Design review of the part built by this model. Coordinates are the model's own, in mm. Coordinates: 2 decimals unless noted, no trailing zeros. Loops run counter-clockwise (first coordinate to the right, second up) from the corner with the lowest first, then second, coordinate; pieces in that order, holes last. Notation, with made-up numbers: (71, 9.25) -> (97, 9.25) arc R21 cw to (97, 19.25) -> close; hole circle Ø4 at (76.25, 58.25). An arc over 180 degrees is marked (long way). Use a Markdown table: item, result. Add a question column.
Q1. For probe 1 along Y at (x, z) = (35, 2.5); probe 2 along Y at (x, z) = (27, 0.75), list the stretches that pass through material, from the lowest coordinate up.
Q2. Clearance check with flat-ended pins moving along their axes: pin 1 Ø3 at (x, y) = (272.72, 11.25) entering from -Z; pin 2 Ø6 at (x, y) = (154, 11.25) entering from +Z. State where each tip first meets the part, or that it passes through.
Q3. Take a section at A-A on z = 2. Write out the cut boundary in (x, y).
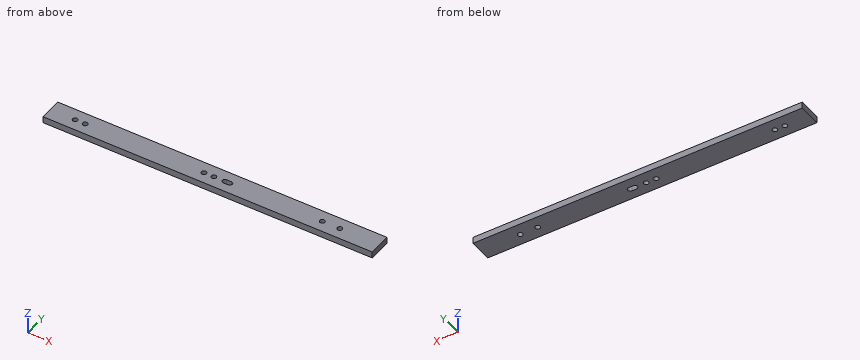
from build123d import *

# Parameters (mm, degrees)
SKETCH_W     = 330
SKETCH_H     = 23
PAD_DEPTH    = 6.5
SKETCH001_R  = 2.5
POCKET_DEPTH = 6.501


with BuildPart() as part:
    # Sketch → Pad (new body)
    with BuildSketch(Plane.XY):
        with Locations((165, 11.5)):
            Rectangle(SKETCH_W, SKETCH_H)
    extrude(amount=PAD_DEPTH)

    # Sketch001 (on Face6 of Pad) → Pocket (cut, through all)
    with BuildSketch(Plane.XY.offset(6.5)):
        with Locations((25, 11.25)):
            Circle(SKETCH001_R)
        with Locations((35, 11.25)):
            Circle(SKETCH001_R)
        with Locations((154, 11.25)):
            Circle(SKETCH001_R)
        with Locations((164, 11.25)):
            Circle(SKETCH001_R)
        with Locations((272.722137, 11.25)):
            Circle(SKETCH001_R)
        with Locations((290.250244, 11.25)):
            Circle(SKETCH001_R)
        with BuildLine():
            ThreePointArc((175, 13.75), (172.5, 11.25), (175, 8.75))
            Line((175, 8.75), (180, 8.75))
            ThreePointArc((180, 8.75), (182.5, 11.25), (180, 13.75))
            Line((175, 13.75), (180, 13.75))
        make_face()
    extrude(amount=-POCKET_DEPTH, mode=Mode.SUBTRACT)


solid = part.part
Answer list:
| question | item | result |
|---|---|---|
| 1 | probe 1 | 0 to 8.75, 13.75 to 23 |
| 1 | probe 2 | 0 to 9.75, 12.75 to 23 |
| 2 | pin 1 | through |
| 2 | pin 2 | z = 6.5 |
| 3 | outline | (0, 0) -> (330, 0) -> (330, 23) -> (0, 23) -> close; hole circle Ø5 at (25, 11.25); hole circle Ø5 at (35, 11.25); hole circle Ø5 at (154, 11.25); hole circle Ø5 at (164, 11.25); hole (175, 8.75) -> (180, 8.75) arc R2.5 ccw to (180, 13.75) -> (175, 13.75) arc R2.5 ccw to start; hole circle Ø5 at (272.72, 11.25); hole circle Ø5 at (290.25, 11.25) |
